```python
from build123d import *

# Parameters (mm, degrees)
ESQUISSE1_W             = 19
ESQUISSE1_H             = 70
ESQUISSE1_R             = 1.7
BOSS_EXTRU_1_DEPTH      = 2
ESQUISSE2_W             = 8
ESQUISSE2_H             = 16
BOSS_EXTRU_2_DEPTH      = 4
ESQUISSE3_R             = 1.4
ENL_V_MAT_EXTRU_1_DEPTH = 4


with BuildPart() as part:
    # Esquisse1 → Boss.-Extru.1 (new body)
    with BuildSketch(Plane.XY):
        with Locations((-2.5, -24.85)):
            Rectangle(ESQUISSE1_W, ESQUISSE1_H)
        Circle(ESQUISSE1_R, mode=Mode.SUBTRACT)
        with Locations((0, -49.7)):
            Circle(ESQUISSE1_R, mode=Mode.SUBTRACT)
    extrude(amount=BOSS_EXTRU_1_DEPTH)

    # Esquisse2 → Boss.-Extru.2 (add)
    with BuildSketch(Plane.ZY.offset(12)):
        with Locations((4, -24.85)):
            Rectangle(ESQUISSE2_W, ESQUISSE2_H)
    extrude(amount=-BOSS_EXTRU_2_DEPTH)

    # Esquisse3 → Enlèv. mat.-Extru.1 (cut)
    with BuildSketch(Plane.ZY.offset(12)):
        with Locations((5, -24.85)):
            Circle(ESQUISSE3_R)
    extrude(amount=-ENL_V_MAT_EXTRU_1_DEPTH, mode=Mode.SUBTRACT)


solid = part.part
```
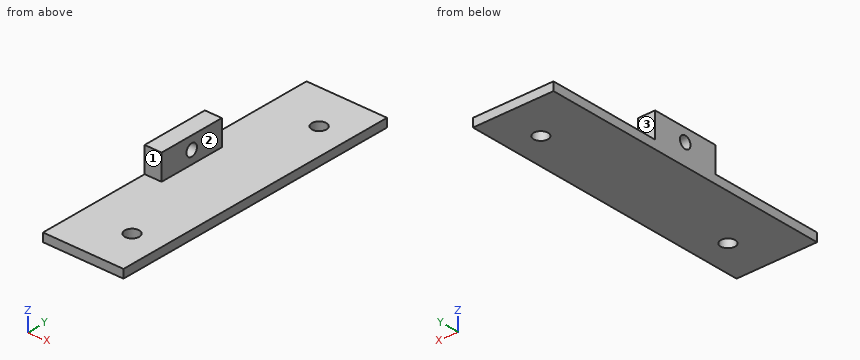
Source: CAD feature listing. Evaluate the final solid. Frame: model axes, mm. Face numbers are marked on the shaded views. A direction names the side the tool comes from. Round coordinates to 2 decimals unless told otherwise and drop trailing zeros. Loops run counter-clockwise (first coordinate to the right, second up) from the corner with the lowest first, then second, coordinate; pieces in that order, holes last.
1. Section query D-D on x = 3.25. Output: boundary loops of the cut face in (y, z).
2. Section query C-C on y = -49.7. Output: boundary loops of the cut face in (x, z), and give its area (3 significant figures).
3. Section query A-A on z = 5. Output: boundary loops of the cut face in (x, y), and give its area (3 significant figures).
4. Ray query, L1, parallel to Y at x = 0, z = 1.55; L2, parallel to Y at x = -10.9, z = 5; L3, parallel to X at y = -32.5, z = 4. Return the intervals inside material, ascending.
5. Contact query for flat-ended pins moving along their axis: pin 1 (4.5 mm diameter, centred on x = -10, z = 4.5, fed in from -Y); pin 2 (2 mm diameter, centred on x = -11, z = 6, fed in from +Y); pin 3 (5 mm diameter, centred on x = -3.5, y = -11, fed in from +Z); pin 4 (3 mm diameter, centred on x = 0, y = -49.7, fed in from +Z). Output: stop coordinate, or through.
6. Section query B-B on y = -24.85. Output: boundary loops of the cut face in (x, z), and give its area (3 significant figures).
7. Access query for the marked faces 1, 2 and 3. Directions: +Z, -Z, +X, -X, +Y, -Y. A direction counts if a zero-diameter tool reaches every point of the face in a straight line with its end or side. Return the directions, or none.
Answers below:
1. outline: (-59.85, 0) - (10.15, 0) - (10.15, 2) - (-59.85, 2) - close
2. outline: (-12, 0) - (-1.7, 0) - (-1.7, 2) - (-12, 2) - close; (1.7, 0) - (7, 0) - (7, 2) - (1.7, 2) - close
2. area: 31.2 mm2
3. outline: (-12, -32.85) - (-8, -32.85) - (-8, -26.25) - (-12, -26.25) - close; (-12, -23.45) - (-8, -23.45) - (-8, -16.85) - (-12, -16.85) - close
3. area: 52.8 mm2
4. L1: y = -59.85 to -51.4, -48 to -1.7, 1.7 to 10.15
4. L2: y = -32.85 to -26.25, -23.45 to -16.85
4. L3: x = -12 to -8
5. pin 1: stops at y = -32.85
5. pin 2: stops at y = -16.85
5. pin 3: stops at z = 2
5. pin 4: passes through
6. outline: (-12, 0) - (7, 0) - (7, 2) - (-8, 2) - (-8, 3.6) - (-12, 3.6) - close; (-12, 6.4) - (-8, 6.4) - (-8, 8) - (-12, 8) - close
6. area: 50.8 mm2
7. face 1: +Z, +X, -X, -Y
7. face 2: +Z, +X, +Y, -Y
7. face 3: +Z, +X, -X, +Y
